Geometry check sheet. Reference: the model listing, model coordinates, mm. Coordinates: 2 decimals unless noted, no trailing zeros. Order: outer loops, then holes, each group sorted by start corner. A loop starts at its lowest first (then second) coordinate and runs counter-clockwise, first axis right, second up. Notation, with made-up numbers: (18.25, 43) - (29.25, 43) arc R25 ccw to (29.25, 71) - close; hole circle Ø7 at (-1, 75.5). An arc over 180 degrees is marked (long way). Return JSON: item names as keys, results as strings. Group by question number.
Item 1: Gauge pin test, flat ends, axial feed: pin 1 (3 mm diameter, centred on x = 8.5, y = 4.5, fed in from +Z); pin 2 (1.8 mm diameter, centred on x = -57, y = 4.5, fed in from -Z); pin 3 (1.8 mm diameter, centred on x = -65.5, y = 2, fed in from -Z). Record the tip position at first contact, or that the pin passes through.
Item 2: Scan lines: probe 1 along Z at (x, y) = (50, 2.45); probe 2 along X at (y, z) = (3.55, -30.75); probe 3 along Z at (x, y) = (0, 3.15). Record each from-to range of solid material in increasing order.
Item 3: Section check C-C on x = 0. Enter the section's corners in (y, z).
Item 4: Section check B-B on z = 23.25. Enter the section's corners in (x, y), then the cut area to 3 significant figures.
Item 5: Section check A-A on x = -50. Enter the section's corners in (y, z).
Item 6: Section check D-D on y = 1.9. Give the number of separate pieces and of enclosed holes in the cut face, then the cut area to 3 significant figures.
from build123d import *

# Parameters (mm, degrees)
BOSS_EXTRUDE2_DEPTH = 6
SKETCH2_R           = 2.5
SKETCH2_R_2         = 12.5
SKETCH2_W           = 25
SKETCH2_H           = 10
CUT_EXTRUDE2_DEPTH  = 6


with BuildPart() as part:
    # Sketch1 → Boss-Extrude2 (new body)
    with BuildSketch(Plane(origin=(0, 0, 0), x_dir=(1, 0, 0), z_dir=(0, 1, 0))):
        Polygon((-62.5, -60), (-54, -60), (-54, -66), (-42, -66), (-42, -60), (-30, -60), (-30, -66), (-18, -66), (-18, -60), (-6, -60), (-6, -66), (6, -66), (6, -60), (18, -60), (18, -66), (30, -66), (30, -60), (42, -60), (42, -66), (54, -66), (54, -60), (62.5, -60), (62.5, -54), (68.5, -54), (68.5, -42), (62.5, -42), (62.5, -30), (68.5, -30), (68.5, -18), (62.5, -18), (62.5, -6), (68.5, -6), (68.5, 6), (62.5, 6), (62.5, 18), (68.5, 18), (68.5, 30), (62.5, 30), (62.5, 42), (68.5, 42), (68.5, 54), (62.5, 54), (62.5, 60), (54, 60), (54, 66), (42, 66), (42, 60), (30, 60), (30, 66), (18, 66), (18, 60), (6, 60), (6, 66), (-6, 66), (-6, 60), (-18, 60), (-18, 66), (-30, 66), (-30, 60), (-42, 60), (-42, 66), (-54, 66), (-54, 60), (-62.5, 60), (-62.5, 54), (-68.5, 54), (-68.5, 42), (-62.5, 42), (-62.5, 30), (-68.5, 30), (-68.5, 18), (-62.5, 18), (-62.5, 6), (-68.5, 6), (-68.5, -6), (-62.5, -6), (-62.5, -18), (-68.5, -18), (-68.5, -30), (-62.5, -30), (-62.5, -42), (-68.5, -42), (-68.5, -54), (-62.5, -54), align=None)
    extrude(amount=BOSS_EXTRUDE2_DEPTH)

    # Sketch2 → Cut-Extrude2 (cut)
    with BuildSketch(Plane(origin=(0, 6, 0), x_dir=(1, 0, 0), z_dir=(0, 1, 0))):
        with Locations((-50, -23.25)):
            Circle(SKETCH2_R)
        with Locations((0, -23.25)):
            Circle(SKETCH2_R_2)
        with Locations((50, -23.25)):
            Circle(SKETCH2_R)
        with Locations((-50, 30.75)):
            Circle(SKETCH2_R)
        with Locations((0, 30.75)):
            Rectangle(SKETCH2_W, SKETCH2_H)
        with Locations((50, 30.75)):
            Circle(SKETCH2_R)
    extrude(amount=-CUT_EXTRUDE2_DEPTH, mode=Mode.SUBTRACT)


solid = part.part
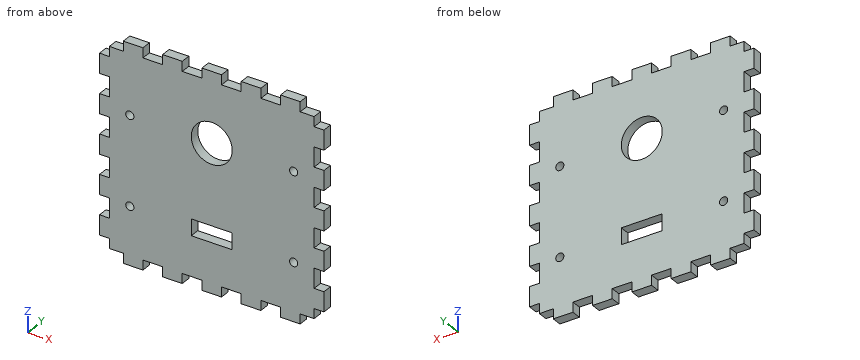
Computed:
{
 "1": {"pin 1": "stops at z = 60", "pin 2": "stops at z = -60", "pin 3": "stops at z = -54"},
 "2": {"probe 1": "z = -66 to -33.25, -28.25 to 20.75, 25.75 to 66", "probe 2": "x = -62.5 to -52.5, -47.5 to -12.5, 12.5 to 47.5, 52.5 to 62.5", "probe 3": "z = -66 to -35.75, -25.75 to 10.75, 35.75 to 66"},
 "3": {"outline": "(0, -66) - (6, -66) - (6, -35.75) - (0, -35.75) - close; (0, -25.75) - (6, -25.75) - (6, 10.75) - (0, 10.75) - close; (0, 35.75) - (6, 35.75) - (6, 66) - (0, 66) - close"},
 "4": {"outline": "(-68.5, 0) - (-52.5, 0) - (-52.5, 6) - (-68.5, 6) - close; (-47.5, 0) - (-12.5, 0) - (-12.5, 6) - (-47.5, 6) - close; (12.5, 0) - (47.5, 0) - (47.5, 6) - (12.5, 6) - close; (52.5, 0) - (68.5, 0) - (68.5, 6) - (52.5, 6) - close", "area": "612 mm²"},
 "5": {"outline": "(0, -66) - (6, -66) - (6, -33.25) - (0, -33.25) - close; (0, -28.25) - (6, -28.25) - (6, 20.75) - (0, 20.75) - close; (0, 25.75) - (6, 25.75) - (6, 66) - (0, 66) - close"},
 "6": {"separate pieces": "1", "enclosed holes": "6", "area": "15,600 mm²"}
}
